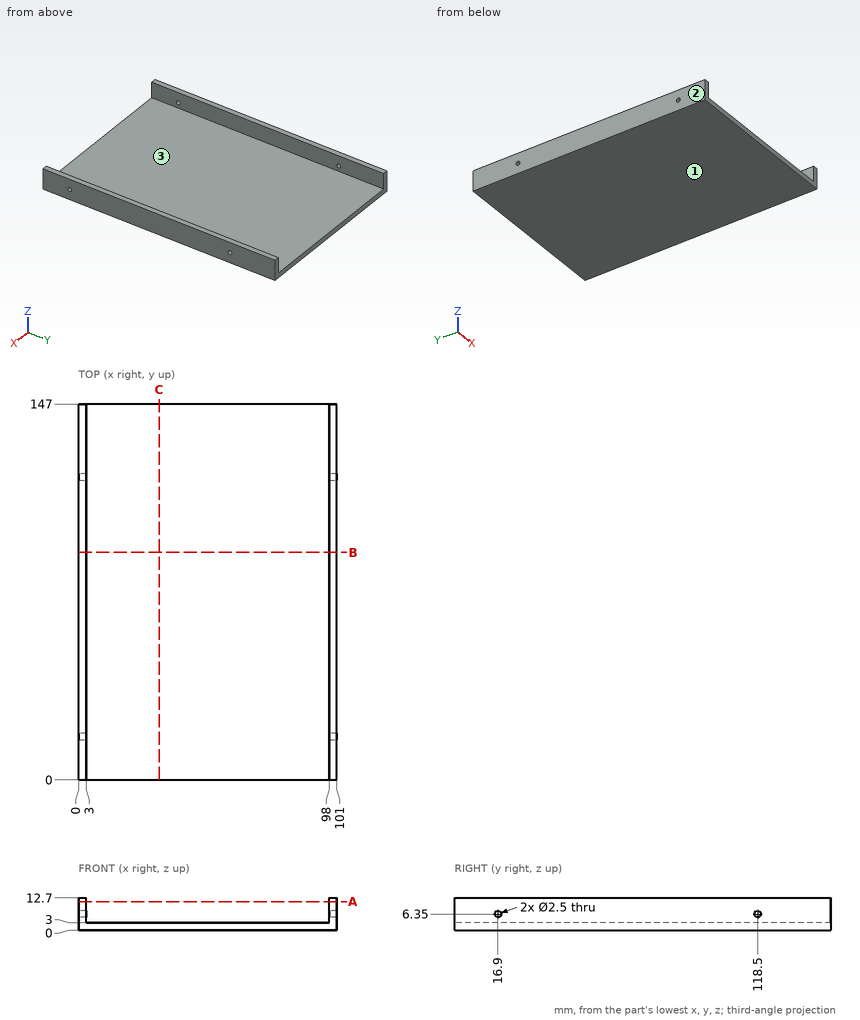
Geometry check sheet. Reference: drawing and pictorial views, mm from the part's lowest x, y, z. Round coordinates to 2 decimals unless told otherwise and drop trailing zeros. Loops run counter-clockwise (first coordinate to the right, second up) from the corner with the lowest first, then second, coordinate; pieces in that order, holes last. Notation, with made-up numbers: (-4, -23.5) - (48, -23.5) arc R26 cw to (48, 6.5) - close; hole circle Ø5 at (34, 30.25). An arc over 180 degrees is marked (long way). Write item = value, one per line. Start each with the question number.
Q1. Release check for a two-part mould opening along X. For the marked faces 1, 2 and 3 record: pulls with the +X half, pulls with the -X half, needs draft (parallel to the pull), parting line crosses it, or undercut.
Q2. Section check A-A (z = 11.25). Record the boundary of the cut face in (x, y), plus the area to 3 significant figures.
Q3. Depth check by flat-ended pin: P1, Ø10, axis at x = 56, y = 38.5, coming from the +Z side; P2, Ø1, axis at y = 25.5, z = 8, coming from the -X side; P3, Ø2, axis at y = 118.5, z = 6.35, coming from the +X side. Enter the tip coordinate at first touch or a pass-through.
Q4. Thickness scan on L1, parallel to X at y = 65.5, z = 5; L2, parallel to Z at x = 0.8, y = 16.9; L3, parallel to Z at x = 5.5, y = 53. Record the ranges inside material, lowest first.
Q5. Section check B-B (y = 89). Record the boundary of the cut face in (x, z).
Q6. Section check C-C (x = 31.5). Record the boundary of the cut face in (y, z), plus the area to 3 significant figures.
Derived:
q1.face_1 = needs draft
q1.face_2 = pulls with the -X half
q1.face_3 = undercut
q2.outline = (0, 0) - (3, 0) - (3, 147) - (0, 147) - close; (98, 0) - (101, 0) - (101, 147) - (98, 147) - close
q2.area = 882 mm^2
q3.P1 = 3
q3.P2 = 0
q3.P3 = through
q4.L1 = 0 to 3, 98 to 101
q4.L2 = 0 to 5.1, 7.6 to 12.7
q4.L3 = 0 to 3
q5.outline = (0, 0) - (101, 0) - (101, 12.7) - (98, 12.7) - (98, 3) - (3, 3) - (3, 12.7) - (0, 12.7) - close
q6.outline = (0, 0) - (147, 0) - (147, 3) - (0, 3) - close
q6.area = 441 mm^2
